Input: part model. Units: mm. Frame: model coordinates. A direction names the side the tool comes from. Round coordinates to 2 decimals unless told otherwise and drop trailing zeros. Write each loop counter-clockwise with the first axis right and the second up, starting at its lowest first coordinate (ties: lowest second). Pieces come first, ordered by that corner, then holes. Notation, with made-up numbers: (35, 52) -> (61, 52) arc R20 ccw to (61, 66) -> close; hole circle Ø5 at (82.25, 20). An arc over 180 degrees is marked (long way). Write item = value, one per line.
```python
from build123d import *

# Parameters (mm, degrees)
SKETCH1_W           = 120
SKETCH1_H           = 250
BOSS_EXTRUDE1_DEPTH = 100
CUT_EXTRUDE4_DEPTH  = 296.999195185
SKETCH3_R           = 25.822682523
CUT_EXTRUDE5_DEPTH  = 295.78805946
CUT_EXTRUDE6_DEPTH  = 50
SKETCH5_R           = 21.439897113
BOSS_EXTRUDE2_DEPTH = 76


with BuildPart() as part:
    # Sketch1 → Boss-Extrude1 (new body)
    with BuildSketch(Plane.XY):
        with Locations((-62.945205479, 125)):
            Rectangle(SKETCH1_W, SKETCH1_H)
    extrude(amount=BOSS_EXTRUDE1_DEPTH)

    # Sketch2 → Cut-Extrude4 (cut, through all)
    with BuildSketch(Plane.XY.offset(100)):
        with BuildLine():
            ThreePointArc((-30.008304656, 92.477893201), (-62.446707823, 126.977893201), (-94.885110989, 92.477893201))
            Line((-94.885110989, 92.477893201), (-94.885110989, 0))
            Line((-94.885110989, 0), (-30.008304656, 0))
            Line((-30.008304656, 0), (-30.008304656, 92.477893201))
        make_face()
        with BuildLine():
            Line((-122.945205479, 250), (-122.945205479, 92.904251347))
            ThreePointArc((-122.945205479, 92.904251347), (-118.821122518, 114.436385128), (-107.294308503, 133.085068837))
            ThreePointArc((-107.294308503, 133.085068837), (-97.704359806, 148.661484818), (-94.358441298, 166.644718124))
            Line((-94.358441298, 166.644718124), (-94.358441298, 250))
            Line((-94.358441298, 250), (-122.945205479, 250))
        make_face()
        with BuildLine():
            ThreePointArc((-16.569647846, 131.918295936), (-7.86521834, 118.575996693), (-2.945205479, 103.424181106))
            Line((-2.945205479, 103.424181106), (-2.945205479, 250))
            Line((-2.945205479, 250), (-28.654722245, 250))
            Line((-28.654722245, 250), (-28.654722245, 164.513670097))
            ThreePointArc((-28.654722245, 164.513670097), (-25.536201958, 147.131873297), (-16.569647846, 131.918295936))
        make_face()
    extrude(amount=-CUT_EXTRUDE4_DEPTH, mode=Mode.SUBTRACT)

    # Sketch3 → Cut-Extrude5 (cut, through all)
    with BuildSketch(Plane(origin=(-2.945205479, 0, 0), x_dir=(0, 0, -1), z_dir=(1, 0, 0))):
        with BuildLine():
            Line((-75.822682523, 117.037988815), (-75.822682523, 250))
            Line((-75.822682523, 250), (-100, 250))
            Line((-100, 250), (-100, 164.513670097))
            Line((-100, 164.513670097), (-100, 131.918295936))
            Line((-100, 131.918295936), (-100, 103.424181106))
            Line((-100, 103.424181106), (-77.711724939, 103.424181106))
            ThreePointArc((-77.711724939, 103.424181106), (-76.297194746, 110.165866843), (-75.822682523, 117.037988815))
        make_face()
        with BuildLine():
            ThreePointArc((-87.942678111, 84.402038305), (-81.787788797, 93.35406738), (-77.711724939, 103.424181106))
            Line((-77.711724939, 103.424181106), (-100, 103.424181106))
            Line((-100, 103.424181106), (-100, 54.589503668))
            ThreePointArc((-100, 54.589503668), (-96.429252241, 70.48984448), (-87.942678111, 84.402038305))
        make_face()
        with BuildLine():
            ThreePointArc((0, 48.834677438), (-50, 1.629363928), (-100, 48.834677438))
            Line((-100, 48.834677438), (-100, 0))
            Line((-100, 0), (0, 0))
            Line((0, 0), (0, 48.834677438))
        make_face()
        with BuildLine():
            Line((0, 103.424181106), (-22.288275061, 103.424181106))
            ThreePointArc((-22.288275061, 103.424181106), (-18.212211203, 93.35406738), (-12.057321889, 84.402038305))
            ThreePointArc((-12.057321889, 84.402038305), (-3.570747759, 70.48984448), (0, 54.589503668))
            Line((0, 54.589503668), (0, 103.424181106))
        make_face()
        with BuildLine():
            Line((0, 250), (-24.177317477, 250))
            Line((-24.177317477, 250), (-24.177317477, 117.037988815))
            ThreePointArc((-24.177317477, 117.037988815), (-23.702805254, 110.165866843), (-22.288275061, 103.424181106))
            Line((-22.288275061, 103.424181106), (0, 103.424181106))
            Line((0, 103.424181106), (0, 131.918295936))
            Line((0, 131.918295936), (0, 164.513670097))
            Line((0, 164.513670097), (0, 250))
        make_face()
        with Locations((-50, 51.712090553)):
            Circle(SKETCH3_R)
    extrude(amount=-CUT_EXTRUDE5_DEPTH, mode=Mode.SUBTRACT)

    # Sketch4 → Cut-Extrude6 (cut)
    with BuildSketch(Plane(origin=(0, 250, 0), x_dir=(1, 0, 0), z_dir=(0, 1, 0))):
        Polygon((-94.358441298, -43.871698339), (-78.810697557, -24.177317477), (-94.358441298, -24.177317477), align=None)
        Polygon((-78.20485695, -75.822682523), (-94.358441298, -59.669098176), (-94.358441298, -75.822682523), align=None)
        Polygon((-28.654722245, -24.177317477), (-45.717868589, -24.177317477), (-28.654722245, -43.871698339), align=None)
        Polygon((-28.654722245, -75.822682523), (-28.654722245, -59.669098176), (-45.717868589, -75.822682523), align=None)
    extrude(amount=-CUT_EXTRUDE6_DEPTH, mode=Mode.SUBTRACT)

    # Sketch5 → Boss-Extrude2 (add)
    with BuildSketch(Plane(origin=(0, 250, 0), x_dir=(1, 0, 0), z_dir=(0, 1, 0))):
        with Locations(Location((-62.112822921, -50, 0), (0, 0, 270))):
            Circle(SKETCH5_R)
    extrude(amount=BOSS_EXTRUDE2_DEPTH)


solid = part.part
```
1) Cut plane A-A (z = 50). Return the cut outline in (x, y), and give its area (3 significant figures).
Solutions:
outline = (-122.95, 1.63) -> (-94.89, 1.63) -> (-94.89, 25.89) -> (-122.95, 25.89) -> close; (-122.95, 77.53) -> (-94.89, 77.53) -> (-94.89, 92.48) arc R32.5 cw (long way) to (-30.01, 92.48) -> (-30.01, 77.53) -> (-2.95, 77.53) -> (-2.95, 103.42) arc R60.5 ccw to (-16.57, 131.92) arc R50 cw to (-28.65, 164.51) -> (-28.65, 250) -> (-40.67, 250) -> (-40.67, 326) -> (-83.55, 326) -> (-83.55, 250) -> (-94.36, 250) -> (-94.36, 166.64) arc R50 cw to (-107.29, 133.09) arc R60.5 ccw to (-122.95, 92.9) -> close; (-30.01, 1.63) -> (-2.95, 1.63) -> (-2.95, 25.89) -> (-30.01, 25.89) -> close
area = 16,100 mm^2
2) Cut plane B-B (x = -99.5). Return the cut outline in (y, z), and give its area (4 significant figures).
Solutions:
outline = (48.83, 0) -> (54.59, 0) arc R50.08 ccw to (84.4, 12.06) arc R50 cw to (117.04, 24.18) -> (144.56, 24.18) -> (144.56, 75.82) -> (117.04, 75.82) arc R50 cw to (84.4, 87.94) arc R50.08 ccw to (54.59, 100) -> (48.83, 100) arc R50.08 ccw to start; hole circle Ø51.65 at (51.71, 50)
area = 8,225 mm^2
3) Line query: L1, parallel to X at y = 82, z = 72; L2, parallel to Y at x = -105, z = 50; L3, parallel to Y at x = -103.25, z = 50. Output: solid intervals per line, ascending. Write a range as from..to.
Solutions:
L1 = -122.95..-94.89, -30.01..-2.95
L2 = 1.63..25.89, 77.53..135.81
L3 = 1.63..25.89, 77.53..138.18
4) Cut plane D-D (y = 298). Return the cut outline in (x, z).
Solutions:
outline = circle Ø42.88 at (-62.11, 50)
5) Cut plane C-C (y = 185). Return the cut outline in (x, z).
Solutions:
outline = (-94.36, 24.18) -> (-28.65, 24.18) -> (-28.65, 75.82) -> (-94.36, 75.82) -> close
6) First-contact query: P1, Ø3, axis at x = -46.5, y = 178, coming from the -Z side; P2, Ø18, axis at x = -36, z = 68, coming from the +Y side; P3, Ø12, axis at x = -56, z = 54.5, coming from the -Y side. Flat tips, straight axial feed; report the tip coordinate or a pass-through.
Solutions:
P1 = 24.18
P2 = 250
P3 = 124.5
7) Access query for faces 4 (the face through (-86.17, 225.35, 67.86)), 5 (the face through (-86.69, 225.35, 34.16)), 6 (the face through (-40.855, 287.468, 47.209)). Directions: +Z, -Z, +X, -X, +Y, -Y. A direction counts if a zero-diameter tool reaches every point of the face in a straight line with its end or side. Return the directions, or none.
Solutions:
face_4 = +Z, -X, +Y
face_5 = -Z, -X, +Y
face_6 = +Y
8) Draft query along X for faces 1 (the face through (-94.885, 27.5, 39.6)), 2 (the face through (-2.945, 74, 72)), 3 (the face through (-34, 200, 71)). Return one class per face: +X half, -X half, draft (parallel to the pull), parting line (faces both ways), or undercut.
Solutions:
face_1 = undercut
face_2 = +X half
face_3 = draft
